Study the drawing (mm; zero at the part's minimum x, y, z) and answer. A direction names the side the tool comes from. Coordinates: 2 decimals unless noted, no trailing zeros. Order: outer loops, then holes, each group sorted by start corner. A loop starts at its lowest first (then second) coordinate and runs counter-clockwise, first axis right, second up. Notation, with made-up numbers: (-7.5, 63) -> (5.5, 63) arc R6 ccw to (5.5, 68) -> close; hole circle Ø10 at (18.5, 89). An arc over 180 degrees is marked (long way). Answer as CSV lines item,"result". Start each with the question number.
Item 1: Which of the six approach directions +Z, -Z, +X, -X, +Y, -Y give full straight-line access (tool end or side, diameter ignored) to the marked faces 4, 5 and 6?
Item 2: For a pull along X with two mould halves and no side action, classify the marked faces 1, 2 and 3 as pulls with the +X half, pulls with the -X half, needs draft (parallel to the pull), parting line crosses it, or undercut.
Item 3: Each of these flat-tipped pins is pushed along its axis until it touches: pin 1 Ø13.5 at (x, z) = (23.5, 32.5) entering from -Y; pin 2 Ø4 at (x, y) = (26.5, 131) entering from +Z; pin 3 Ø1 at (x, y) = (24.5, 154) entering from -Z. Where does it stop, or does it pass through?
Item 4: Section A-A (x = 50.5) is taken. Write down the section's boundary in (y, z).
Item 5: Section B-B (z = 50) is taken. Write down the section's boundary in (x, y), then the cut area to 4 significant figures.
Item 6: Section C-C (y = 385) is taken. Write down the section's boundary in (x, z).
Item 7: Straight lines are drawn through the part: L1, parallel to X at y = 363.5, z = 82; L2, parallel to Y at x = 57, z = 50; L3, parallel to Y at x = 52.5, z = 41.5. For each, find the intervals that lie inside material, in ascending order.
Item 8: Section D-D (x = 21) is taken. Write down the section's boundary in (y, z).
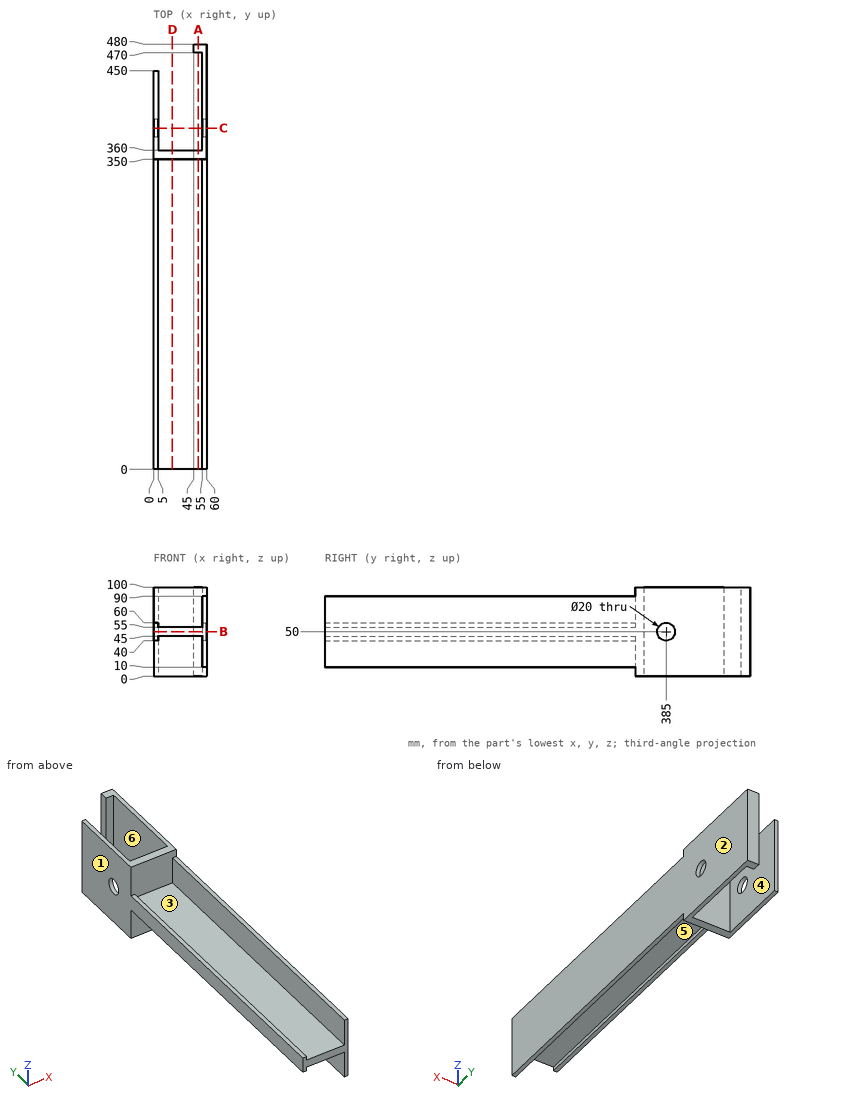
Checked values:
1,face 4,"+Z, -Z, +Y"
1,face 5,"-Z, -Y"
1,face 6,"+Z, -Z"
2,face 1,"pulls with the -X half"
2,face 2,"pulls with the +X half"
2,face 3,"undercut"
3,pin 1,"stops at y = 350"
3,pin 2,"stops at z = 55"
3,pin 3,"stops at z = 45"
4,outline,"(0, 45) -> (350, 45) -> (350, 0) -> (360, 0) -> (360, 100) -> (350, 100) -> (350, 55) -> (0, 55) -> close; (470, 0) -> (480, 0) -> (480, 100) -> (470, 100) -> close"
5,outline,"(0, 0) -> (60, 0) -> (60, 375) -> (55, 375) -> (55, 360) -> (5, 360) -> (5, 375) -> (0, 375) -> close; (0, 395) -> (5, 395) -> (5, 450) -> (0, 450) -> close; (45, 470) -> (55, 470) -> (55, 395) -> (60, 395) -> (60, 480) -> (45, 480) -> close"
5,area,"22,550 mm^2"
6,outline,"(0, 0) -> (5, 0) -> (5, 40) -> (0, 40) -> close; (0, 60) -> (5, 60) -> (5, 100) -> (0, 100) -> close; (55, 0) -> (60, 0) -> (60, 40) -> (55, 40) -> close; (55, 60) -> (60, 60) -> (60, 100) -> (55, 100) -> close"
7,L1,"x = 0 to 5, 55 to 60"
7,L2,"y = 0 to 375, 395 to 480"
7,L3,"y = 350 to 360, 470 to 480"
8,outline,"(0, 45) -> (350, 45) -> (350, 0) -> (360, 0) -> (360, 100) -> (350, 100) -> (350, 55) -> (0, 55) -> close"
